Part model, mm, in its own coordinate system. A direction names the side the tool comes from. Round coordinates to 2 decimals unless told otherwise and drop trailing zeros. Write each loop counter-clockwise with the first axis right and the second up, starting at its lowest first coordinate (ties: lowest second). Pieces come first, ordered by that corner, then holes. Notation, with made-up numbers: M 50.5,55 L 90.5,55 A26 cw 90.5,85 Z; hole C 23,-23 d9. An arc over 180 degrees is marked long. Use a Markdown table: item, result. Add a question column.
1) Drop flat-ended pins along their axis: P1, Ø1.5, axis at y = 2.5, z = 2, coming from the -X side (3 decimals); P2, Ø0.6, axis at y = 3.5, z = -2.5, coming from the +X side; P3, Ø0.6, axis at x = 0, y = 5, coming from the -Z side. Give the stop position or say it passes through.
2) Slice it at A-A on z = -2. Write the cut outline in (x, y) (3 decimals), plus the area to 3 significant figures.
3) Slice it at C-C on x = 1.85. Write the cut outline in (y, z) (3 decimals), plus the area to 3 significant figures.
4) Which spindle directions (+Z, -Z, +X, -X, +Y, -Y) get a long thin tool onto all of the face, cutting with end or side? Do faces 1 (the face through (0, 3, -2.265)), 2 (the face through (-1, 1.613, -2)), 3 (the face through (1, 0.762, 0)). Say none if no direction does.
5) Slice it at B-B on y = 6.25. Give the number of separate pieces and of enclosed holes in the cut face, plus the area to 3 significant figures.
6) Two-plate mould, pull along Z, no slides. Class faces 4 (the face through (-1, 1, 0.708)), 5 (the face through (-1, 1.613, 2)), 6 (the face through (0, 6.5, -2.9)): released by +Z, released by -Z, zero draft, split by the parting line, or undercut.
7) Wall check: probe 1 along Z at (x, y) = (-0.2, 5) (3 decimals); probe 2 along Z at (x, y) = (1.85, 4.5); probe 3 along Z at (x, y) = (-0.35, 5.5). Give the ranges that are in metal, low to high.
```python
from build123d import *

# Parameters (mm, degrees)
SKETCH1_W                  = 4.5
SKETCH1_H                  = 5.8
EXTRUDE1_DEPTH             = 7
SKETCH10_W                 = 1.2954
SKETCH10_H                 = 0.635
SKETCH10_W_2               = 1.1938
CUT_EXTRUDE7_DEPTH         = 6.8
CUT_EXTRUDE13_DEPTH        = 5.5
SKETCH3_W                  = 1.0668
SKETCH3_H                  = 1.0668
MATING_SIDE_CHAMFERS_DEPTH = 0.508
MATING_SIDE_CHAMFERS_TAPER = 45
SKETCH18_W                 = 5.8
SKETCH18_H                 = 7
POLARIZING_KEYWAY_DEPTH    = 0.7874
SKETCH4_W                  = 0.8668
SKETCH4_H                  = 0.8668
TERMINAL_HOLES_DEPTH       = 8
SKETCH14_W                 = 0.8668
SKETCH14_H                 = 0.8668
TERMINAL_CUTOUT_DEPTH      = 5.73
RAMP1_DEPTH                = 0.7874
TERMINALLOCK_CUTOUT_DEPTH  = 0.9398
SKETCH20_W                 = 0.249
SKETCH20_H                 = 2.7051
CUT_EXTRUDE16_DEPTH        = 0.9398
LPATTERN2_COUNT            = 2
LPATTERN2_PITCH            = 2


with BuildPart() as part:
    # Sketch1 → Extrude1 (new body)
    with BuildSketch(Plane(origin=(0, 0, 0), x_dir=(1, 0, 0), z_dir=(0, 1, 0))):
        Rectangle(SKETCH1_W, SKETCH1_H)
    extrude(amount=EXTRUDE1_DEPTH)

    # Sketch10 → Cut-Extrude7 (cut, through all)
    with BuildSketch(Plane(origin=(0, 4.9, 2.9), x_dir=(1, 0, 0), z_dir=(0, 0, -1))):
        Polygon((-0.5948, 4.9), (0.0656, 4.138), (2.25, 4.138), (2.25, 4.9), align=None)
        Polygon((-2.25, -1.2214), (-1.615, -0.1038), (-1.615, 4.9), (-2.25, 4.9), align=None)
        with Locations((-1.6023, -1.7825)):
            Rectangle(SKETCH10_W, SKETCH10_H)
        with Locations((1.6531, -1.7825)):
            Rectangle(SKETCH10_W_2, SKETCH10_H)
    extrude(amount=CUT_EXTRUDE7_DEPTH, mode=Mode.SUBTRACT)

    # Sketch17 → Cut-Extrude13 (cut, through all)
    with BuildSketch(Plane(origin=(2.25, 0, 0), x_dir=(0, 0, -1), z_dir=(1, 0, 0))):
        Polygon((-2.9, 0), (-2.265, 0), (-2.265, 5.0038), (-2.9, 6.1214), align=None)
        Polygon((2.9, 0), (2.265, 0), (2.265, 5.0038), (2.9, 6.1214), align=None)
    extrude(amount=-CUT_EXTRUDE13_DEPTH, mode=Mode.SUBTRACT)

    # Sketch3 → Mating Side Chamfers (cut)
    with BuildSketch(Plane.XZ.offset(-0.762)):
        with Locations((0.699, 1)):
            Rectangle(SKETCH3_W, SKETCH3_H)
    mating_side_chamfers = extrude(amount=-MATING_SIDE_CHAMFERS_DEPTH, taper=MATING_SIDE_CHAMFERS_TAPER, mode=Mode.SUBTRACT)

    # Sketch18 → Polarizing Keyway (cut)
    with BuildSketch(Plane(origin=(2.25, 0, 0), x_dir=(0, 0, -1), z_dir=(1, 0, 0))):
        with Locations((0, 3.5)):
            Rectangle(SKETCH18_W, SKETCH18_H)
        Polygon((0.7874, 0.762), (0.7874, 5.5014), (-0.7874, 5.5014), (-0.7874, 0.762), (-1.4478, 0.762), (-1.7526, 1.0668), (-1.7526, 6.365), (1.7526, 6.365), (1.7526, 1.0668), (1.4478, 0.762), align=None, mode=Mode.SUBTRACT)
    extrude(amount=-POLARIZING_KEYWAY_DEPTH, mode=Mode.SUBTRACT)

    # Sketch4 → Terminal Holes (cut, through all)
    with BuildSketch(Plane.XZ):
        with Locations((0.699, 1)):
            Rectangle(SKETCH4_W, SKETCH4_H)
    terminal_holes = extrude(amount=-TERMINAL_HOLES_DEPTH, mode=Mode.SUBTRACT)

    # Sketch14 → Terminal Cutout (cut)
    with BuildSketch(Plane(origin=(0, 7, 0), x_dir=(-1, 0, 0), z_dir=(0, 1, 0))):
        Polygon((1.6108, 0.42074158), (1.6108, 1.57925842), (1.179, 1.57925842), (1.179, 1.7747), (-0.7768, 1.7747), (-0.7768, 1.5715), (-1.2086, 1.5715), (-1.2086, 1), (-1.2086, 0.4285), (-0.7768, 0.4285), (-0.7768, 0.2253), (1.179, 0.2253), (1.179, 0.42074158), align=None)
        with Locations((-0.699, 1)):
            Rectangle(SKETCH14_W, SKETCH14_H, mode=Mode.SUBTRACT)
    terminal_cutout = extrude(amount=-TERMINAL_CUTOUT_DEPTH, mode=Mode.SUBTRACT)

    # Sketch11 → Ramp1 (add)
    with BuildSketch(Plane.XY.offset(2.265)):
        Polygon((1.4626, 2.77196042), (1.4626, 2.032), (1.6658, 2.2352), (1.6658, 2.56876042), align=None)
    ramp1 = extrude(amount=-RAMP1_DEPTH)

    # Sketch19 → TerminalLock Cutout (cut)
    with BuildSketch(Plane.ZY.offset(1.615)):
        Polygon((0.365, 4.318), (0.365, 2.2352), (1.635, 2.2352), (1.635, 4.318), (2.016, 4.318), (2.016, 1.6129), (1.2921, 1.6129), (1.2921, 0.5842), (0.7079, 0.5842), (0.7079, 1.6129), (-0.016, 1.6129), (-0.016, 4.318), align=None)
    terminallock_cutout = extrude(amount=-TERMINALLOCK_CUTOUT_DEPTH, mode=Mode.SUBTRACT)

    # Sketch20 → Cut-Extrude16 (cut)
    with BuildSketch(Plane.ZY.offset(1.615)):
        with Locations((2.1405, 2.96545)):
            Rectangle(SKETCH20_W, SKETCH20_H)
        with Locations((-2.1405, 2.96545)):
            Rectangle(SKETCH20_W, SKETCH20_H)
    extrude(amount=-CUT_EXTRUDE16_DEPTH, mode=Mode.SUBTRACT)

    # LPattern2: Mating Side Chamfers, Terminal Holes, Terminal Cutout, TerminalLock Cutout ×2
    with Locations(*[(0, 0, -i * LPATTERN2_PITCH) for i in range(1, LPATTERN2_COUNT)]):
        add(mating_side_chamfers, mode=Mode.SUBTRACT)
        add(terminal_holes, mode=Mode.SUBTRACT)
        add(terminal_cutout, mode=Mode.SUBTRACT)
        add(terminallock_cutout, mode=Mode.SUBTRACT)

    # Mirror1: Ramp1 across plane
    add(ramp1.mirror(Plane.XY))


solid = part.part
```
Entries:
| question | item | result |
|---|---|---|
| 1 | P1 | stops at x = -1.615 |
| 1 | P2 | stops at x = 1.46 |
| 1 | P3 | stops at z = -2.43 |
| 2 | outline | M -2.25,6.121 L -1.615,5.004 L -1.615,4.318 L -0.675,4.318 L -0.675,1.613 L -1.615,1.613 L -1.615,0 L -0.595,0 L 0.066,0.762 L 1.463,0.762 L 1.463,2.032 L 1.666,2.235 L 1.666,2.569 L 1.463,2.772 L 1.463,6.365 L 1.056,6.365 L 1.056,7 L -0.955,7 L -0.955,6.365 L -2.25,6.365 Z |
| 2 | area | 17.6 mm^2 |
| 3 | outline | M 0.762,-1.448 L 1.067,-1.753 L 6.365,-1.753 L 6.365,1.753 L 1.067,1.753 L 0.762,1.448 L 0.762,0.787 L 5.501,0.787 L 5.501,-0.787 L 0.762,-0.787 Z |
| 3 | area | 12.1 mm^2 |
| 4 | face 1 | -Z, +X, -X, -Y |
| 4 | face 2 | +Z, -Z, -X |
| 4 | face 3 | +Z, -Z, +X, -Y |
| 5 | separate pieces | 1 |
| 5 | enclosed holes | 2 |
| 5 | area | 16.2 mm^2 |
| 6 | face 4 | undercut |
| 6 | face 5 | zero draft |
| 6 | face 6 | released by -Z |
| 7 | probe 1 | z = -2.265 to -1.775, -0.225 to 0.225, 1.775 to 2.265 |
| 7 | probe 2 | z = -1.75 to -0.79, 0.79 to 1.75 |
| 7 | probe 3 | z = -2.55 to -1.77, -0.23 to 0.23, 1.77 to 2.55 |
